Design review of the part built by this model. Coordinates are the model's own, in mm. A direction names the side the tool comes from. Give positions to 0.01 mm unless a question says otherwise; leave off trailing zeros. Loops run counter-clockwise (first coordinate to the right, second up) from the corner with the lowest first, then second, coordinate; pieces in that order, holes last. Notation, with made-up numbers: M 3,78.25 L 48,78.25 A13 cw 48,102.25 Z; hole C 60.25,-1.5 d3. An arc over 180 degrees is marked long. Use one line per item in the form item = value. Start each with the question number.
from build123d import *

# Parameters (mm, degrees)
F1_DEPTH     = 10
F3_DEPTH     = 25
F4_R         = 3
F5_DEPTH     = 12.5
F6_R         = 4.99999
F7_R         = 11.2793724654
F8_W         = 12.0593691245
F8_H         = 3
F9_DEPTH     = 25
F10_T4_DEPTH = 35.7540736123
F10_T9_DEPTH = 35.7540736123


# Not quite as in the source:
# - a fillet or chamfer that OpenCascade refuses, or shapes differently, is made with other operations: its cross-section is extruded or revolved along the edge and cut away or added
# - a fillet or chamfer is up to 0.001 mm smaller than in the source, because OpenCascade refuses the exact size


with BuildPart() as f1:
    # F0 (on Front) → F1 (new body)
    with BuildSketch(Plane.XZ):
        Polygon((-29.8706907779, 13), (-29.8706907779, 0), (-29.8706907779, -13), (23.6637946218, -7), (23.6637946218, 0), (23.6637946218, 7), align=None)
    extrude(amount=F1_DEPTH)

    # F2 (on face) → F3 (cut)
    with BuildSketch(Plane.XZ.offset(10)):
        with BuildLine():
            ThreePointArc((-25.3706907779, 0), (-19.8706907779, -5.5), (-14.3706907779, 0))
            ThreePointArc((-14.3706907779, 0), (-19.8706907779, 5.5), (-25.3706907779, 0))
        make_face()
    extrude(amount=-F3_DEPTH, mode=Mode.SUBTRACT)

    # F4 (on Top) → F5 (cut, symmetric)
    with BuildSketch(Plane.XY):
        with Locations((17.7213400602, -4.9999998882)):
            Circle(F4_R)
    extrude(amount=F5_DEPTH, both=True, mode=Mode.SUBTRACT)

    # F6 (radius 5 in the source; OpenCascade refuses exactly that, so slightly less here)
    f6_edges = [f1.edges().sort_by_distance(p)[0] for p in [
        (23.663795, -10, 0),
        (23.663795, 0, 0),
    ]]
    fillet(f6_edges, radius=F6_R)

    # F7
    f7_edges = [f1.edges().sort_by_distance(p)[0] for p in [
        (-29.870691, -5, 13),
        (-29.870691, -5, -13),
    ]]
    fillet(f7_edges, radius=F7_R)

    # F8 (on Front) → F9 (cut)
    with BuildSketch(Plane.XZ):
        Polygon((12.0786419138, 3), (12.0786419138, 0), (24.1380110383, 0), (24.2066532373, 3), align=None)
        with Locations((18.1083264761, -1.5)):
            Rectangle(F8_W, F8_H)
        Polygon((25.2308808267, -17.6116619259), (24.1380110383, -7), (12.0786419138, -7), (12.0786419138, -17.6116619259), align=None)
        Polygon((12.0786419138, 14.7170173004), (12.0786419138, 7), (24.2066532373, 7), (23.395627737, 15.3522975743), align=None)
    extrude(amount=F9_DEPTH, mode=Mode.SUBTRACT)

    # F10: chamfer of 5 on 2 edges, made by hand


with BuildPart() as f10_tool2:
    # F10_s3 → F10_t4 (new body)
    with BuildSketch(Plane.XZ.offset(22.8770368062)):
        Polygon((12.0786419138, -3.29843251), (7.1097524238, -8.8553321741), (12.0786419138, -8.29843251), align=None)
    extrude(amount=-F10_T4_DEPTH)

    split(bisect_by=Plane.XY.offset(-7), keep=Keep.BOTTOM)


with BuildPart() as f1_1:
    add(f1.part)

    # F10_t1: cut F10_tool2
    add(f10_tool2.part, mode=Mode.SUBTRACT)


with BuildPart() as f10_tool7:
    # F10_s8 → F10_t9 (new body)
    with BuildSketch(Plane.XZ.offset(-12.8770368062)):
        Polygon((7.1097524238, 8.8553321741), (12.0786419138, 3.29843251), (12.0786419138, 8.29843251), align=None)
    extrude(amount=F10_T9_DEPTH)

    split(bisect_by=Plane.XY.offset(7), keep=Keep.TOP)


with BuildPart() as f1_2:
    add(f1_1.part)

    # F10_t6: cut F10_tool7
    add(f10_tool7.part, mode=Mode.SUBTRACT)


solid = f1_2.part
Q1. The part is to be moulded in two halves that separate along X. For faces 1 (the flat face through (-4.9, -4.9, 10.2)), 2 (the flat face through (15, -3, -3)), 3 (the cylindrical face through (-25.365, -5.07, 0.242)), say which applies: pulls with the +X half, pulls with the -X half, needs draft (parallel to the pull), parting line crosses it, or undercut.
Q2. For faces 4 (the flat face through (14.7, -6, -7)), 5 (the flat face through (15, -3, 3)), 6 (the cylindrical face through (22.16, -1.426, -4.972)), 7 (the flat face through (14, -5, 7)), 8 (the flat face through (-6, -10, 0)), list the 3-axis set-ups (+Z, -Z, +X, -X, +Y, -Y) from which the entire face can be reached by the end or side of a thin tool; tool diameter is ignored.
Q3. Wall thickness on probe 1 along X at (y, z) = (-3.75, 4.5); probe 2 along Z at (x, y) = (12.5, -1.5); probe 3 along X at (y, z) = (-8, 0.25) (3 decimals): over which ranges is each line inside the solid? List them lowest first.
Q4. Take a section at B-B on y = -4.5. Give the boundary of the cut face in (x, z).
Q5. Clearance check with flat-ended pins moving along their axes: pin 1 Ø1.8 at (y, z) = (-7, 1) entering from +X; pin 2 Ø6 at (y, z) = (-2.5, 4.5) entering from +X; pin 3 Ø2 at (x, y) = (-15, -2) entering from -Z; pin 4 Ø3 at (x, y) = (9.5, -7) entering from -Z. State where each tip first meets the part, or that it passes through.
Q6. Take a section at A-A on z = -4.25. State how many separate pieces and enclosed holes the cut face has, plus the area to 3 significant figures.
Q7. Take a section at C-C on x = 16.5. Give the boundary of the cut face in (y, z), plus the area to 3 significant figures.
Response values:
q1.face_1 = pulls with the +X half
q1.face_2 = needs draft
q1.face_3 = undercut
q2.face_4 = -Z, +X, +Y, -Y
q2.face_5 = +X, +Y, -Y
q2.face_6 = +Z, -Z, +X, +Y
q2.face_7 = +Z, +X, +Y, -Y
q2.face_8 = +Z, -Z, +X, -X, -Y
q3.probe_1 = -29.09 to -23.03, -16.71 to 14.99, 20.45 to 23.51
q3.probe_2 = -7 to -3, 3 to 7
q3.probe_3 = -29.871 to -25.365, -14.376 to 12.079
q4.outline = M -29.87,-0.39 A11.28 ccw -17.34,-11.6 L 7.11,-8.86 L 8.77,-7 L 14.76,-7 L 14.76,-3 L 12.08,-3 L 12.08,3 L 14.76,3 L 14.76,7 L 8.77,7 L 7.11,8.86 L -17.34,11.6 A11.28 ccw -29.87,0.39 Z; M 20.68,-7 L 23.64,-7 L 23.64,-3 L 20.68,-3 Z; M 20.68,3 L 23.64,3 L 23.64,7 L 20.68,7 Z; hole C -19.87,0 d11
q5.pin_1 = 12.08
q5.pin_2 = 23.66
q5.pin_3 = -11.45
q5.pin_4 = -7.86
q6.separate_pieces = 2
q6.enclosed_holes = 1
q6.area = 420 mm^2
q7.outline = M -10,-7 L -7.74,-7 L -7.74,-3 L -10,-3 Z; M -10,3 L -7.74,3 L -7.74,7 L -10,7 Z; M -2.26,-7 L 0,-7 L 0,-3 L -2.26,-3 Z; M -2.26,3 L 0,3 L 0,7 L -2.26,7 Z
q7.area = 36.2 mm^2
